Autodesk Inventor part; units mm, degrees
ref_plane "YZ Plane" through (0, 0, 0) normal (1, 0, 0) x (0, 1, 0)
ref_plane "XZ Plane" through (0, 0, 0) normal (0, 1, 0) x (-1, 0, 0)
ref_plane "XY Plane" through (0, 0, 0) normal (0, 0, 1) x (1, 0, 0)
sketch "Sketch1" plane through (0, 0, 0) normal (0, 1, 0) x (-1, 0, 0)
  circle A0 centre (0, 0) radius 7
  circle A1 centre (0, 0) radius 8
  dimension "d0" = 14
  dimension "d1" = 1
extrude "Extrusion1" add sketch "Sketch1" along normal blind 10.5
sketch "Sketch2" plane through (0, 0, 0) normal (0, -1, 0) x (1, 0, 0)
  circle A0 centre (0, 0) radius 8
extrude "Extrusion2" add sketch "Sketch2" against normal blind 0.5
sketch "Sketch4" plane through (0, 10.5, 0) normal (0, 1, 0) x (1, 0, 0)
  circle A0 centre (-10, 0) radius 1.25
  circle A1 centre (-10, 0) radius 2.5
  point P0 (0, 0)
  dimension "d6" = 5
  dimension "d7" = 2.5
  dimension "d8" = 10
extrude "Extrusion3" add sketch "Sketch4" against normal up to surface (10.5 mm away)
pattern_circular "Circular Pattern1" count 4 over 360 about axis through (0, 0, 0) along (0, 1, 0) of "Extrusion3"
fillet "Fillet1" radius 1 8 edges at (7.8875, 5.25, -1.3369) (7.8875, 5.25, 1.3369) (1.3369, 5.25, 7.8875) (-1.3369, 5.25, 7.8875) (-7.8875, 5.25, 1.3369) (-7.8875, 5.25, -1.3369) (-1.3369, 5.25, -7.8875) (1.3369, 5.25, -7.8875)
properties part number "PDMS_insert"
Can you work these out from the model? Positions are in its coordinate system, mm. A direction names the side the tool comes from. Give positions to 0.01 mm unless a question says otherwise; leave off trailing zeros. Loops run counter-clockwise (first coordinate to the right, second up) from the corner with the lowest first, then second, coordinate; pieces in that order, holes last. Notation, with made-up numbers: M 15,-19 L 70,-19 A20 cw 70,-7 Z; hole C -40,26.25 d8. An arc over 180 degrees is marked long. Use one line per item in the form item = value. Start each with the question number.
(1) I'm going to push flat-ended pins straight in: P1, Ø4, axis at x = -7.5, y = 7.5, coming from the +Z side; P2, Ø1.5, axis at y = 8, z = -4.5, coming from the +X side; P3, Ø4, axis at x = 3, z = -2.5, coming from the +Y side; P4, Ø2, axis at x = 0, z = 10, coming from the -Y side. Where does each tip first touch, or does it pass through?
(2) On a 3-axis mill with a long thin cutter (end or side, diameter ignored), from which of +Z, -Z, +X, -X, +Y, -Y can I reach the whole of each face in a straight line? I mean faces 4 (the cylindrical face through (-11.25, 5.32, -0.05)), 5 (the cylindrical face through (-6.466, 5.43, 2.681)). Say none if no direction works.
(3) I want a section at B-B, the plane x = -10. Write out the boundary of the cut face in (y, z), and give its area (4 significant figures).
(4) I want a section at A-A, the plane z = -10. Write out the boundary of the cut face in (x, y).
(5) I want a section at D-D, the plane z = 3.75. Write out the boundary of the cut face in (x, y), and give its area (3 significant figures).
(6) I want a section at C-C, the plane x = 0. Write out the boundary of the cut face in (y, z), and give its area (3 significant figures).
(7) Thinking about a two-plate mould opening in Z: for faces 1 (the cylindrical face through (-0.05, 5.32, 11.25)), 2 (the cylindrical face through (-5.691, 5.177, -5.623)), 3 (the cylindrical face through (5.691, 5.177, 5.623)), which applies, released by +Z, released by -Z, zero draft, split by the parting line, or undercut?
(8) Please list where these lines run through material, in increasing order: line 1 (Z direction, x = -10, y = 3.75); line 2 (Z direction, x = 0.25, y = 1).
Worked out:
q1.P1 = 5.81
q1.P2 = 7.07
q1.P3 = 0.5
q1.P4 = through
q2.face_4 = +Y, -Y
q2.face_5 = +Y
q3.outline = M 0,-2.5 L 10.5,-2.5 L 10.5,-1.25 L 0,-1.25 Z; M 0,1.25 L 10.5,1.25 L 10.5,2.5 L 0,2.5 Z
q3.area = 26.25 mm²
q4.outline = M -2.5,0 L -1.25,0 L -1.25,10.5 L -2.5,10.5 Z; M 1.25,0 L 2.5,0 L 2.5,10.5 L 1.25,10.5 Z
q5.outline = M -7.07,0 L 7.07,0 L 7.07,10.5 L 5.91,10.5 L 5.91,0.5 L -5.91,0.5 L -5.91,10.5 L -7.07,10.5 Z
q5.area = 30.2 mm²
q6.outline = M 0,-12.5 L 10.5,-12.5 L 10.5,-11.25 L 0,-11.25 Z; M 0,-8.75 L 10.5,-8.75 L 10.5,-7 L 0.5,-7 L 0.5,7 L 10.5,7 L 10.5,8.75 L 0,8.75 Z; M 0,11.25 L 10.5,11.25 L 10.5,12.5 L 0,12.5 Z
q6.area = 70.0 mm²
q7.face_1 = undercut
q7.face_2 = released by -Z
q7.face_3 = released by +Z
q8.line_1 = -2.5 to -1.25, 1.25 to 2.5
q8.line_2 = -12.49 to -11.22, -8.78 to -7, 7 to 8.78, 11.22 to 12.49
